```python
from build123d import *

# Parameters (mm, degrees)
EXTRUDE_1_DEPTH = 15
FILLET_1_R      = 5.1
FILLET_2_R      = 5
FILLET_3_R      = 5
FILLET_4_R      = 5


with BuildPart() as part:
    # 스케치1 → 보스-돌출1 (new body)
    with BuildSketch(Plane.XY):
        Polygon((0, 0), (32, 0), (52, 28.562960135), (35.616959114, 40.034488862), (25.08969668, 25), (0, 25), align=None)
    extrude(amount=EXTRUDE_1_DEPTH)

    # 필렛1
    fillet_1_edges = [part.edges().sort_by_distance(p)[0] for p in [
        (35.616959114, 40.034488862, 7.5),
    ]]
    fillet(fillet_1_edges, radius=FILLET_1_R)

    # 필렛2
    fillet_2_edges = [part.edges().sort_by_distance(p)[0] for p in [
        (32, 0, 7.5),
    ]]
    fillet(fillet_2_edges, radius=FILLET_2_R)

    # 필렛3
    fillet_3_edges = [part.edges().sort_by_distance(p)[0] for p in [
        (0, 25, 7.5),
    ]]
    fillet(fillet_3_edges, radius=FILLET_3_R)

    # 필렛4
    fillet_4_edges = [part.edges().sort_by_distance(p)[0] for p in [
        (52, 28.562960135, 7.5),
    ]]
    fillet(fillet_4_edges, radius=FILLET_4_R)


solid = part.part
```
Verification items for the finished model (mm, model axes). A direction names the side the tool comes from. Give positions to 0.01 mm unless a question says otherwise; leave off trailing zeros. Order: outer loops, then holes, each group sorted by start corner. A loop starts at its lowest first (then second) coordinate and runs counter-clockwise, first axis right, second up. Notation, with made-up numbers: M -28,-17.5 L 19,-17.5 A17 cw 19,-8.5 Z; hole C -38,-34 d11. An arc over 180 degrees is marked long. Return JSON: item names as keys, results as strings. Group by question number.
1) Access from +Z, -Z, +X, -X, +Y, -Y to the whole of each face (thin tool, end or side, straight path). Record for faces 1 (the face through (15, 25, 7)), 2 (the face through (31.736, 0.581, 7.605)).
2) Section check B-B on x = 22. Record the cut outline in (y, z), and give its area (3 significant figures).
3) Go/stop test with flat-tipped pins: pin 1 Ø4.5 at (x, z) = (16, 11) entering from +Y; pin 2 Ø8 at (x, y) = (36, 10) entering from -Z; pin 3 Ø2 at (y, z) = (9, 7.5) entering from +X; pin 4 Ø6 at (y, z) = (9, 10.5) entering from +X. Record where each tip stops, or that it passes through.
4) Section check A-A on z = 9.75. Record the cut outline in (x, y).
5) Section check C-C on y = 27. Record the cut outline in (x, z), and give its area (3 significant figures).
6) Scan lines: line 1 (Y direction, x = 10.5, z = 9.5); line 2 (Y direction, x = 34, z = 6.75); line 3 (X direction, y = 17.5, z = 9.75). Record each from-to range of solid material in increasing order.
Answer block:
{
 "1": {"face 1": "+Z, -Z, -X, +Y", "face 2": "+Z, -Z, +X, -Y"},
 "2": {"outline": "M 0,0 L 25,0 L 25,15 L 0,15 Z", "area": "375 mm^2"},
 "3": {"pin 1": "stops at y = 25", "pin 2": "stops at z = 0", "pin 3": "stops at x = 39", "pin 4": "stops at x = 40.4"},
 "4": {"outline": "M 0,0 L 29.4,0 A5 ccw 33.49,2.13 L 49.13,24.47 A5 ccw 47.9,31.43 L 39.79,37.11 A5.1 ccw 32.69,35.86 L 25.09,25 L 5,25 A5 ccw 0,20 Z"},
 "5": {"outline": "M 26.49,0 L 50.03,0 L 50.03,15 L 26.49,15 Z", "area": "353 mm^2"},
 "6": {"line 1": "y = 0 to 25", "line 2": "y = 2.86 to 37.15", "line 3": "x = 0 to 44.25"}
}
